Solid Edge part; units mm, degrees
sketch "Sketch1" plane through (0, 0, 0) normal (0, -1, 0) x (1, 0, 0)
  line L0 (-75.229, -48.7494) -> (54.771, -48.7494)
  line L1 (54.771, -48.7494) -> (54.771, 51.2506)
  line L2 (54.771, 51.2506) -> (-75.229, 51.2506)
  line L3 (-75.229, 51.2506) -> (-75.229, -48.7494)
  dimension "D1" = 75.229
  dimension "D2" = 54.771
extrude "Protrusion1" add sketch "Sketch1" against normal blind 10
sketch "Sketch2" plane through (24.771, 0, 1.2506) normal (0, -1, 0) x (1, 0, 0)
  circle A0 centre (-65, 0) radius 12.5
  dimension "D1" = 65
extrude "Cutout1" cut sketch "Sketch2" against normal through all
sketch "Sketch3" plane through (-15.229, 10, 1.2506) normal (0, 1, 0) x (-1, 0, 0)
  circle A0 centre (-25, -25) radius 5
  circle A1 centre (-25, 25) radius 5
  circle A2 centre (-55, -25) radius 5
  circle A3 centre (-55, 25) radius 5
extrude "Cutout2" cut sketch "Sketch3" against normal through all
properties material "Aluminum, 6061-T6"
Input: part model. Units: mm. Frame: model coordinates. Give positions to 0.01 mm unless a question says otherwise; leave off trailing zeros. Order: outer loops, then holes, each group sorted by start corner. A loop starts at its lowest first (then second) coordinate and runs counter-clockwise, first axis right, second up. Notation, with made-up numbers: M 9.5,-7 L 15.5,-7 A23 ccw 15.5,15 Z; hole C 4.5,35 d3. An arc over 180 degrees is marked long. One line per question, with ' | ' between items. Start each with the question number.
1. First-contact query: pin 1 Ø9 at (x, z) = (39.77, 26.25) entering from +Y; pin 2 Ø13 at (x, z) = (9.77, 26.25) entering from +Y. Flat tips, straight axial feed; report the tip coordinate or a pass-through.
2. Material intervals for probe 1 along X at (y, z) = (1.75, 26); probe 2 along X at (y, z) = (1.5, -26.5); probe 3 along Z at (x, y) = (11, 7.5), sorted ascending. Write a range as [from, to].
3. Section query C-C (y = 5.75). Return the cut outline in (x, z), and give its area (3 significant figures).
4. Section query B-B (z = -26). Return the cut outline in (x, y), and give its area (3 significant figures).
5. Section query A-A (z = -2). Return the cut outline in (x, y), and give its area (3 significant figures).
6. Pull-direction query (X, two-part tool) for faces 1 (the face through (-75.229, 5, 2)), 2 (the face through (13.456, 5.07, 29.63)), 3 (the face through (-11, 5, -48.749)); classes: released by +X, released by -X, zero draft, split by the parting line, or undercut.
Here are the results:
1) pin 1: through | pin 2: y = 10
2) probe 1: [-75.23, 4.78], [14.76, 34.78], [44.76, 54.77] | probe 2: [-75.23, 5.6], [13.95, 35.6], [43.95, 54.77] | probe 3: [-48.75, -28.6], [-18.9, 21.4], [31.1, 51.25]
3) outline: M -75.23,-48.75 L 54.77,-48.75 L 54.77,51.25 L -75.23,51.25 Z; hole C -40.23,1.25 d25; hole C 9.77,-23.75 d10; hole C 9.77,26.25 d10; hole C 39.77,-23.75 d10; hole C 39.77,26.25 d10 | area: 12,200 mm²
4) outline: M -75.23,0 L 5.31,0 L 5.31,10 L -75.23,10 Z; M 14.24,0 L 35.31,0 L 35.31,10 L 14.24,10 Z; M 44.24,0 L 54.77,0 L 54.77,10 L 44.24,10 Z | area: 1,120 mm²
5) outline: M -75.23,0 L -52.3,0 L -52.3,10 L -75.23,10 Z; M -28.16,0 L 54.77,0 L 54.77,10 L -28.16,10 Z | area: 1,060 mm²
6) face 1: released by -X | face 2: undercut | face 3: zero draft
